```python
from build123d import *

# Parameters (mm, degrees)
BOSS_EXTRUDE1_DEPTH = 0.5
SKETCH2_R           = 1.8
SKETCH2_R_2         = 0.5
BOSS_EXTRUDE2_DEPTH = 0.5
FILLET2_START       = 0.5
FILLET2_2_DEPTH     = 0.5
FILLET3_R           = 1


with BuildPart() as part:
    # Sketch1 → Boss-Extrude1 (new body)
    with BuildSketch(Plane(origin=(0, 0, 0), x_dir=(1, 0, 0), z_dir=(0, 1, 0))):
        with BuildLine():
            Line((-3.5, 0), (-2.5, 0))
            ThreePointArc((-2.5, 0), (0, 2.5), (2.5, 0))
            Line((2.5, 0), (3.5, 0))
            ThreePointArc((3.5, 0), (0, -3.5), (-3.5, 0))
        make_face()
    extrude(amount=BOSS_EXTRUDE1_DEPTH)

    # Sketch2 → Boss-Extrude2 (add)
    with BuildSketch(Plane(origin=(0, 0.5, 0), x_dir=(1, 0, 0), z_dir=(0, 1, 0))):
        with Locations(Location((0, 0, 0), (0, 0, 270))):
            Circle(SKETCH2_R)
        with Locations(Location((0, 0, 0), (0, 0, 270))):
            Circle(SKETCH2_R_2, mode=Mode.SUBTRACT)
    extrude(amount=BOSS_EXTRUDE2_DEPTH)

    # Fillet2: read off the stored shape, not the designer's step
    # Fillet2 outline → Fillet2 (revolve)
    with BuildSketch(Plane.XY):
        with BuildLine():
            ThreePointArc((3.122875656, 0.5), (2.415768875, 0.629171307), (1.8, 1))
            Line((1.8, 1), (1.8, 0.5))
            Line((1.8, 0.5), (3.122875656, 0.5))
        make_face()
    revolve(axis=Axis((0, 0, 0), (0, 1, 0)))

    # Fillet2 2 outline → Fillet2 2 (cut)
    with BuildSketch(Plane(origin=(0, 0, 0), x_dir=(1, 0, 0), z_dir=(0, 1, 0)).offset(FILLET2_START)):
        with BuildLine():
            ThreePointArc((-2.5, 0), (0, 2.5), (2.5, 0))
            Line((2.5, 0), (5, 0))
            Line((5, 0), (5, 5))
            Line((5, 5), (-5, 5))
            Line((-5, 5), (-5, 0))
            Line((-5, 0), (-2.5, 0))
        make_face()
    extrude(amount=FILLET2_2_DEPTH, mode=Mode.SUBTRACT)

    # Fillet3
    fillet3_edges = [part.edges().sort_by_distance(p)[0] for p in [
        (-1.8, 1, 0),
    ]]
    fillet(fillet3_edges, radius=FILLET3_R)


solid = part.part
```
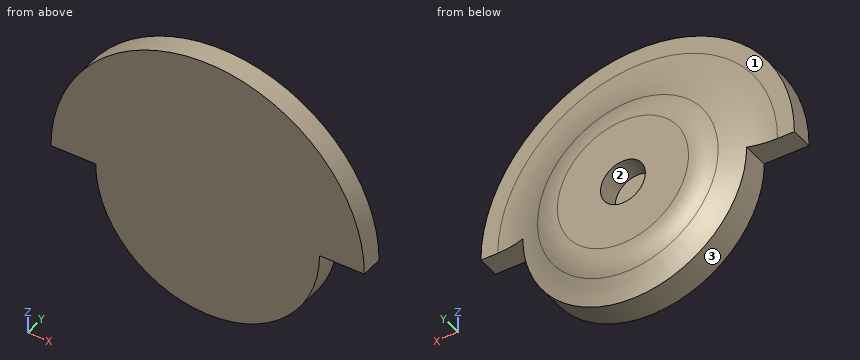
CAD build for the part. Positions are in the model's coordinates, mm. Face numbers are marked on the shaded views. Coordinates: 2 decimals unless noted, no trailing zeros. Write each loop counter-clockwise with the first axis right and the second up, starting at its lowest first coordinate (ties: lowest second). Pieces come first, ordered by that corner, then holes.
(1) Cut at A-A, the plane y = 0.3. List the corners of the cut face in (x, z), and give its area (3 significant figures).
(2) Flat gauge pins, fed straight in: pin 1 (0.8 mm diameter, centred on x = 0, z = 0, fed in from +Y); pin 2 (3 mm diameter, centred on x = -0.5, z = 2.5, fed in from +Y). Where does each tip first touch, or does it go through?
(3) Drill centre lines: probe 1 along Y at (x, z) = (0.5, 3); probe 2 along X at (y, z) = (0.8, 0); probe 3 along X at (y, z) = (0.75, 0). Where is each one in solid material? Low to high.
(4) Two-plate mould, pull along X, no slides. Class the marked faces 1, 2 and 3: +X half, -X half, draft (parallel to the pull), parting line (faces both ways), or undercut.
Geometry says:
1. outline: (-3.5, 0) - (-2.5, 0) arc R2.5 ccw to (2.5, 0) - (3.5, 0) arc R3.5 ccw to start
1. area: 29.1 mm2
2. pin 1: stops at y = 0.5
2. pin 2: stops at y = 1
3. probe 1: y = 0 to 0.5
3. probe 2: x = -2.07 to -0.5, 0.5 to 2.07
3. probe 3: x = -2.15 to -0.5, 0.5 to 2.15
4. face 1: draft
4. face 2: undercut
4. face 3: parting line
